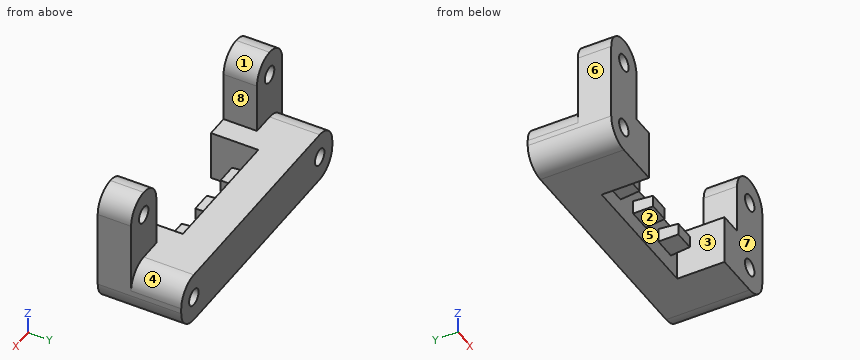
from build123d import *

# Parameters (mm, degrees)
BOSS_EXTRUDE1_DEPTH           = 9
SKETCH2_W                     = 4
SKETCH2_H                     = 2.5
BOSS_EXTRUDE2_DEPTH           = 3.5
BOSS_EXTRUDE2_DRAFT           = 3
BOSS_EXTRUDE2_PROFILE_2_DEPTH = 3.5
BOSS_EXTRUDE2_PROFILE_2_DRAFT = 3
BOSS_EXTRUDE2_PROFILE_3_DEPTH = 3.5
BOSS_EXTRUDE2_PROFILE_3_DRAFT = 3
SKETCH4_W                     = 8
SKETCH4_H                     = 6
BOSS_EXTRUDE4_DEPTH           = 13
SKETCH3_R                     = 1.5
CUT_EXTRUDE1_DEPTH            = 55.890800686
FILLET1_R                     = 4


with BuildPart() as part:
    # Sketch1 → Boss-Extrude1 (new body)
    with BuildSketch(Plane.XY):
        Polygon((0, 0), (12, 0), (12, 8.5), (36, 8.5), (36, 0), (48, 0), (48, 15), (0, 15), align=None)
    extrude(amount=BOSS_EXTRUDE1_DEPTH)


with BuildPart() as boss_extrude2_tool:
    # Sketch2 → Boss-Extrude2 (with draft: the straight prism first)
    with BuildSketch(Plane(origin=(0, 8.5, 0), x_dir=(-1, 0, 0), z_dir=(0, -1, 0))):
        with Locations((-16, -4.5)):
            Rectangle(SKETCH2_W, SKETCH2_H)
    extrude(amount=BOSS_EXTRUDE2_DEPTH)
    # Boss-Extrude2: the draft: its side faces are tilted about the plane it starts from
    boss_extrude2_sides = [boss_extrude2_tool.faces().sort_by_distance(p)[0] for p in [
        (14, 6.75, 4.5),
        (16, 6.75, 3.25),
        (18, 6.75, 4.5),
        (16, 6.75, 5.75),
    ]]
    draft(boss_extrude2_sides, Plane(origin=(0, 8.5, 0), x_dir=(-1, 0, 0), z_dir=(0, -1, 0)), BOSS_EXTRUDE2_DRAFT)


with BuildPart() as part_1:
    add(part.part)

    # Boss-Extrude2: add boss_extrude2_tool
    add(boss_extrude2_tool.part)


with BuildPart() as boss_extrude2_profile_2_tool:
    # Sketch2 → Boss-Extrude2 profile 2 (with draft: the straight prism first)
    with BuildSketch(Plane(origin=(0, 8.5, 0), x_dir=(-1, 0, 0), z_dir=(0, -1, 0))):
        with Locations((-24, -4.5)):
            Rectangle(SKETCH2_W, SKETCH2_H)
    extrude(amount=BOSS_EXTRUDE2_PROFILE_2_DEPTH)
    # Boss-Extrude2 profile 2: the draft: its side faces are tilted about the plane it starts from
    boss_extrude2_profile_2_sides = [boss_extrude2_profile_2_tool.faces().sort_by_distance(p)[0] for p in [
        (22, 6.75, 4.5),
        (24, 6.75, 3.25),
        (26, 6.75, 4.5),
        (24, 6.75, 5.75),
    ]]
    draft(boss_extrude2_profile_2_sides, Plane(origin=(0, 8.5, 0), x_dir=(-1, 0, 0), z_dir=(0, -1, 0)), BOSS_EXTRUDE2_PROFILE_2_DRAFT)


with BuildPart() as part_2:
    add(part_1.part)

    # Boss-Extrude2 profile 2: add boss_extrude2_profile_2_tool
    add(boss_extrude2_profile_2_tool.part)


with BuildPart() as boss_extrude2_profile_3_tool:
    # Sketch2 → Boss-Extrude2 profile 3 (with draft: the straight prism first)
    with BuildSketch(Plane(origin=(0, 8.5, 0), x_dir=(-1, 0, 0), z_dir=(0, -1, 0))):
        with Locations((-32, -4.5)):
            Rectangle(SKETCH2_W, SKETCH2_H)
    extrude(amount=BOSS_EXTRUDE2_PROFILE_3_DEPTH)
    # Boss-Extrude2 profile 3: the draft: its side faces are tilted about the plane it starts from
    boss_extrude2_profile_3_sides = [boss_extrude2_profile_3_tool.faces().sort_by_distance(p)[0] for p in [
        (30, 6.75, 4.5),
        (32, 6.75, 3.25),
        (34, 6.75, 4.5),
        (32, 6.75, 5.75),
    ]]
    draft(boss_extrude2_profile_3_sides, Plane(origin=(0, 8.5, 0), x_dir=(-1, 0, 0), z_dir=(0, -1, 0)), BOSS_EXTRUDE2_PROFILE_3_DRAFT)


with BuildPart() as part_3:
    add(part_2.part)

    # Boss-Extrude2 profile 3: add boss_extrude2_profile_3_tool
    add(boss_extrude2_profile_3_tool.part)

    # Sketch4 → Boss-Extrude4 (add)
    with BuildSketch(Plane.XY.offset(9)):
        with Locations((4, 3)):
            Rectangle(SKETCH4_W, SKETCH4_H)
        with Locations((44, 3)):
            Rectangle(SKETCH4_W, SKETCH4_H)
    extrude(amount=BOSS_EXTRUDE4_DEPTH)

    # Sketch3 → Cut-Extrude1 (cut, through all)
    with BuildSketch(Plane(origin=(0, 15, 0), x_dir=(1, 0, 0), z_dir=(0, 1, 0))):
        with Locations(Location((4, -4.5, 0), (0, 0, 270))):
            Circle(SKETCH3_R)
        with Locations(Location((44, -4.5, 0), (0, 0, 270))):
            Circle(SKETCH3_R)
        with Locations(Location((4, -17.5, 0), (0, 0, 270))):
            Circle(SKETCH3_R)
        with Locations(Location((44, -17.5, 0), (0, 0, 270))):
            Circle(SKETCH3_R)
    extrude(amount=-CUT_EXTRUDE1_DEPTH, mode=Mode.SUBTRACT)

    # Fillet1
    fillet1_edges = [part_3.edges().sort_by_distance(p)[0] for p in [
        (40, 3, 22),
        (48, 3, 22),
        (48, 7.5, 0),
        (48, 10.5, 9),
        (0, 3, 22),
        (8, 3, 22),
        (0, 7.5, 0),
        (0, 10.5, 9),
    ]]
    fillet(fillet1_edges, radius=FILLET1_R - 0.0001)  # a hair under: the kernel refuses the full size


solid = part_3.part
Part model, mm, in its own coordinate system. Face numbers are marked on the shaded views. A direction names the side the tool comes from. Give positions to 0.01 mm unless a question says otherwise; leave off trailing zeros. Order: outer loops, then holes, each group sorted by start corner. A loop starts at its lowest first (then second) coordinate and runs counter-clockwise, first axis right, second up. Notation, with made-up numbers: (51, 63.5) - (98, 63.5) arc R23 cw to (98, 80.5) - close; hole circle Ø3 at (51.25, 40.25). An arc over 180 degrees is marked (long way). One line per question, with ' | ' between items.
1. Pull direction X, two halves, no side cores. Call the marked faces 6, 7 and 8: +X half, -X half, draft (parallel to the pull), parting line (faces both ways), or undercut.
Filled in:
face 6: -X half | face 7: draft | face 8: undercut
2. Drop flat-ended pins along their axis: P1, Ø2.5, axis at x = 44, z = 15.5, coming from the +Y side; P2, Ø4, axis at x = 21.5, y = 9.5, coming from the +Z side; P3, Ø2.5, axis at x = 21.5, z = 6, coming from the -Y side. Give the stop position or say it passes through.
Filled in:
P1: y = 6 | P2: z = 9 | P3: y = 5
3. Which spindle directions (+Z, -Z, +X, -X, +Y, -Y) get a long thin tool onto all of the face, cutting with end or side? Do the marked faces 1, 2, 3, 4 and 5. Say none if no direction does.
Filled in:
face 1: +Z, +Y, -Y | face 2: -Z, -Y | face 3: +Z, -Z, -Y | face 4: +Z, +X, +Y | face 5: -Y
4. Band-saw the part on B-B on z = 12.75. List the corners of the cut face in (x, y).
Filled in:
outline: (0, 0) - (8, 0) - (8, 6) - (0, 6) - close; (40, 0) - (48, 0) - (48, 6) - (40, 6) - close
5. Band-saw the part on A-A on y = 3.25. Give the number of separate pieces and of enclosed holes in the cut face, then the cut area to 3 significant figures.
Filled in:
separate pieces: 2 | enclosed holes: 4 | area: 375 mm²
6. Drill centre lines: probe 1 along X at (y, z) = (2.5, 17.5); probe 2 along X at (y, z) = (3.5, 4.5); probe 3 along X at (y, z) = (10, 4.5). Where is each one in solid material? Low to high.
Filled in:
probe 1: 0 to 2.5, 5.5 to 8, 40 to 42.5, 45.5 to 48 | probe 2: 0 to 2.5, 5.5 to 12, 36 to 42.5, 45.5 to 48 | probe 3: 0 to 2.5, 5.5 to 42.5, 45.5 to 48
7. Band-saw the part on C-C on y = 14. List the corners of the cut face in (x, z).
Filled in:
outline: (0, 4) arc R4 ccw to (4, 0) - (44, 0) arc R4 ccw to (48, 4) - (48, 5) arc R4 ccw to (44, 9) - (4, 9) arc R4 ccw to (0, 5) - close; hole circle Ø3 at (4, 4.5); hole circle Ø3 at (44, 4.5)
8. Band-saw the part on D-D on z = 17.5. List the corners of the cut face in (x, y), then the cut area to 3 significant figures.
Filled in:
outline: (0, 0) - (2.5, 0) - (2.5, 6) - (0, 6) - close; (5.5, 0) - (8, 0) - (8, 6) - (5.5, 6) - close; (40, 0) - (42.5, 0) - (42.5, 6) - (40, 6) - close; (45.5, 0) - (48, 0) - (48, 6) - (45.5, 6) - close | area: 60.0 mm²
